from build123d import *

# Parameters (mm, degrees)
SKETCH_1_R      = 34
SKETCH_1_R_2    = 3
EXTRUDE_1_DEPTH = 4
SKETCH_1_3_R    = 3
SKETCH_1_3_R_2  = 1.5
EXTRUDE_2_DEPTH = 2
SKETCH_2_R      = 5
EXTRUDE_3_DEPTH = 2
EXTRUDE_4_DEPTH = 3


with BuildPart() as part:
    # Sketch 1 → Extrude 1 (new body)
    with BuildSketch(Plane(origin=(0, 0, 0), x_dir=(1, 0, 0), z_dir=(0, 1, 0))):
        Circle(SKETCH_1_R)
        with Locations((-22, 0)):
            Circle(SKETCH_1_R_2, mode=Mode.SUBTRACT)
        with Locations((0, -22)):
            Circle(SKETCH_1_R_2, mode=Mode.SUBTRACT)
        with Locations((22, 0)):
            Circle(SKETCH_1_R_2, mode=Mode.SUBTRACT)
        with Locations((0, 22)):
            Circle(SKETCH_1_R_2, mode=Mode.SUBTRACT)
    extrude(amount=EXTRUDE_1_DEPTH)

    # Sketch 1_3 → Extrude 2 (add)
    with BuildSketch(Plane(origin=(0, 0, 0), x_dir=(1, 0, 0), z_dir=(0, 1, 0))):
        with Locations((0, 22)):
            Circle(SKETCH_1_3_R)
        with Locations((0, 22)):
            Circle(SKETCH_1_3_R_2, mode=Mode.SUBTRACT)
        with Locations((22, 0)):
            Circle(SKETCH_1_3_R)
        with Locations((22, 0)):
            Circle(SKETCH_1_3_R_2, mode=Mode.SUBTRACT)
        with Locations((0, -22)):
            Circle(SKETCH_1_3_R)
        with Locations((0, -22)):
            Circle(SKETCH_1_3_R_2, mode=Mode.SUBTRACT)
        with Locations((-22, 0)):
            Circle(SKETCH_1_3_R)
        with Locations((-22, 0)):
            Circle(SKETCH_1_3_R_2, mode=Mode.SUBTRACT)
    extrude(amount=EXTRUDE_2_DEPTH)

    # Sketch 2 → Extrude 3 (add)
    with BuildSketch(Plane(origin=(0, 4, 0), x_dir=(1, 0, 0), z_dir=(0, 1, 0))):
        Circle(SKETCH_2_R)
    extrude(amount=EXTRUDE_3_DEPTH)

    # Sketch 3 → Extrude 4 (add)
    with BuildSketch(Plane(origin=(0, 6, 0), x_dir=(1, 0, 0), z_dir=(0, 1, 0))):
        with BuildLine():
            Line((-4.330127, 2.5), (4.330127, 2.5))
            ThreePointArc((4.330127, 2.5), (5, 0), (4.330127, -2.5))
            Line((4.330127, -2.5), (-4.330127, -2.5))
            ThreePointArc((-4.330127, -2.5), (-5, 0), (-4.330127, 2.5))
        make_face()
    extrude(amount=EXTRUDE_4_DEPTH)


solid = part.part
Could you check a few things on this model? Use its own coordinates, in mm. A direction names the side the tool comes from. Give positions to 0.01 mm unless a question says otherwise; leave off trailing zeros. Order: outer loops, then holes, each group sorted by start corner. A loop starts at its lowest first (then second) coordinate and runs counter-clockwise, first axis right, second up. Notation, with made-up numbers: (42.25, 63) - (73.25, 63) arc R14 ccw to (73.25, 85) - close; hole circle Ø8 at (-35.75, 7.5). An arc over 180 degrees is marked (long way). One line per question, with ' | ' between items. Start each with the question number.
Item 1: I want a section at C-C on x = 22. Write out the boundary of the cut face in (y, z).
Item 2: For faces 1 (the flat face through (0, 6, -3)), 2 (the cylindrical face through (19, 3, 0)), 3 (the cylindrical face through (-0.195, 0.986, 20.513)), 4 (the flat face through (0, 6, 3)), which set-ups out of +Z, -Z, +X, -X, +Y, -Y let a thin tool reach every point of the face, with its end or its side?
Item 3: I'm going to push flat-ended pins straight in: pin 1 Ø4 at (x, z) = (22, 0) entering from +Y; pin 2 Ø1.2 at (x, z) = (1.5, 4) entering from +Y; pin 3 Ø4 at (y, z) = (2, 12.5) entering from +X; pin 4 Ø4 at (x, z) = (0, -22) entering from -Y. Where does each tip first touch, or does it pass through?
Item 4: I want a section at B-B on x = 0. Write out the boundary of the cut face in (y, z), then the cut area to 3 significant figures.
Item 5: I want a section at D-D on z = -22. Write out the boundary of the cut face in (x, y), then the cut area to 3 significant figures.
Item 6: I want a section at A-A on z = 0. Write out the boundary of the cut face in (x, y).
Item 7: Thinking about a two-plate mould opening in Z: for faces 5 (the flat face through (0, 7, 2.5)), 6 (the flat face through (-20.7, 2, 1.3)), 7 (the flat face through (0, 9, 0)), 8 (the flat face through (0, 7, -2.5)), which applies, pulls with the +Z half, pulls with the -Z half, needs draft (parallel to the pull), parting line crosses it, or undercut?
Item 8: I need wall thicknesses on probe 1 along X at (y, z) = (1.6, 0); probe 2 along X at (y, z) = (3.35, 0). Which ranges of each line are inside material? Lowest first, please. Write a range as [from, to].
Verdict:
1) outline: (0, -25.92) - (4, -25.92) - (4, -3) - (2, -3) - (2, -1.5) - (0, -1.5) - close; (0, 1.5) - (2, 1.5) - (2, 3) - (4, 3) - (4, 25.92) - (0, 25.92) - close
2) face 1: -Z, +X, -X, +Y | face 2: +Y | face 3: +Y, -Y | face 4: +Z, +X, -X, +Y
3) pin 1: y = 2 | pin 2: y = 6 | pin 3: x = 32.34 | pin 4: y = 0
4) outline: (0, -34) - (4, -34) - (4, -25) - (2, -25) - (2, -23.5) - (0, -23.5) - close; (0, -20.5) - (2, -20.5) - (2, -19) - (4, -19) - (4, -5) - (6, -5) - (6, -2.5) - (9, -2.5) - (9, 2.5) - (6, 2.5) - (6, 5) - (4, 5) - (4, 19) - (2, 19) - (2, 20.5) - (0, 20.5) - close; (0, 23.5) - (2, 23.5) - (2, 25) - (4, 25) - (4, 34) - (0, 34) - close | area: 271 mm^2
5) outline: (-25.92, 0) - (-1.5, 0) - (-1.5, 2) - (-3, 2) - (-3, 4) - (-25.92, 4) - close; (1.5, 0) - (25.92, 0) - (25.92, 4) - (3, 4) - (3, 2) - (1.5, 2) - close | area: 189 mm^2
6) outline: (-34, 0) - (-23.5, 0) - (-23.5, 2) - (-25, 2) - (-25, 4) - (-34, 4) - close; (-20.5, 0) - (20.5, 0) - (20.5, 2) - (19, 2) - (19, 4) - (5, 4) - (5, 9) - (-5, 9) - (-5, 4) - (-19, 4) - (-19, 2) - (-20.5, 2) - close; (23.5, 0) - (34, 0) - (34, 4) - (25, 4) - (25, 2) - (23.5, 2) - close
7) face 5: pulls with the +Z half | face 6: undercut | face 7: needs draft | face 8: pulls with the -Z half
8) probe 1: [-34, -23.5], [-20.5, 20.5], [23.5, 34] | probe 2: [-34, -25], [-19, 19], [25, 34]
